The model under review builds one solid part; all positions refer to its coordinate system, in mm. A direction names the side the tool comes from. Coordinates: 2 decimals unless noted, no trailing zeros. Write each loop counter-clockwise with the first axis right and the second up, starting at its lowest first coordinate (ties: lowest second). Pieces come first, ordered by that corner, then holes. Notation, with made-up numbers: (87.5, 42.5) - (93.5, 42.5) arc R31 ccw to (93.5, 67.5) - close; hole circle Ø2 at (-38, 55). An arc over 180 degrees is marked (long way). Put each result on its own line as item: value.
from build123d import *

# Parameters (mm, degrees)
BASPROSKE_W                         = 6.35
BASPROSKE_H                         = 26.19375
TOOTHCUT_DEPTH                      = 7.35
BORSKE_R                            = 6.35
BORE_DEPTH                          = 50.8000508
SKETCH1_R                           = 23.8125
CUT_EXTRUDE1_DEPTH                  = 3.2512
F_9_64_0_14063_DIAMETER_HOLE1_D     = 3.572002
F_9_64_0_14063_DIAMETER_HOLE1_DEPTH = 9.525
F_9_64_0_14063_DIAMETER_HOLE1_TIP   = 1.073137666


with BuildPart() as part:
    # BasProSke → Base-Revolve (revolve)
    with BuildSketch(Plane(origin=(0, 0, 0), x_dir=(1, 0, 0), z_dir=(0, 1, 0))):
        with Locations((3.175, 13.096875)):
            Rectangle(BASPROSKE_W, BASPROSKE_H)
    revolve(axis=Axis((-10, 0, 0), (1, 0, 0)))

    # TooCutSke → ToothCut (cut, through all)
    with BuildSketch(Plane(origin=(0, 0, 0), x_dir=(0, 0, -1), z_dir=(1, 0, 0))):
        with BuildLine():
            ThreePointArc((0.33374141, 24.394417139), (0, 24.3967), (-0.33374141, 24.394417139))
            ThreePointArc((-0.33374141, 24.394417139), (-0.642437388, 25.31332079), (-1.03730144, 26.19862272))
            ThreePointArc((-1.03730144, 26.19862272), (0, 26.21915), (1.03730144, 26.19862272))
            ThreePointArc((1.03730144, 26.19862272), (0.642437388, 25.31332079), (0.33374141, 24.394417139))
        make_face()
    extrude(amount=TOOTHCUT_DEPTH, mode=Mode.SUBTRACT)

    # BorSke → Bore (cut, symmetric)
    with BuildSketch(Plane(origin=(0, 0, 0), x_dir=(0, 0, -1), z_dir=(1, 0, 0))):
        Circle(BORSKE_R)
    extrude(amount=BORE_DEPTH, both=True, mode=Mode.SUBTRACT)

    # Sketch1 → Cut-Extrude1 (cut)
    with BuildSketch(Plane(origin=(6.35, 0, 0), x_dir=(0, 0, -1), z_dir=(1, 0, 0))):
        Circle(SKETCH1_R)
    extrude(amount=-CUT_EXTRUDE1_DEPTH, mode=Mode.SUBTRACT)

    # 9/64 (0.14063) Diameter Hole1
    with Locations(Plane(origin=(3.0988, 0, 0), x_dir=(0, 0, -1), z_dir=(1, 0, 0))):
        with Locations((0, 9.779), (0, 19.05), (7.290119387, 17.599905094), (13.470384182, 13.470384182), (17.599905094, 7.290119387), (19.05, 0), (17.599905094, -7.290119387), (13.470384182, -13.470384182), (7.290119387, -17.599905094), (0, -19.05), (-7.290119387, -17.599905094), (-13.470384182, -13.470384182), (-17.599905094, -7.290119387), (-19.05, 0), (-17.599905094, 7.290119387), (-13.470384182, 13.470384182), (-7.290119387, 17.599905094), (6.914797213, 6.914797213), (9.779, 0), (6.914797213, -6.914797213), (0, -9.779), (-6.914797213, -6.914797213), (-9.779, 0), (-6.914797213, 6.914797213)):
            Hole(F_9_64_0_14063_DIAMETER_HOLE1_D / 2, depth=F_9_64_0_14063_DIAMETER_HOLE1_DEPTH)
            with Locations((0, 0, -(F_9_64_0_14063_DIAMETER_HOLE1_DEPTH + F_9_64_0_14063_DIAMETER_HOLE1_TIP / 2))):  # 118° drill point
                Cone(0, F_9_64_0_14063_DIAMETER_HOLE1_D / 2, F_9_64_0_14063_DIAMETER_HOLE1_TIP, mode=Mode.SUBTRACT)


solid = part.part
1. Consider section C-C on z = -10. State the section outline as (x, y) points, plus the area to 3 significant figures.
Determined:
outline: (0, -24.21) - (6.35, -24.21) - (6.35, -21.61) - (3.1, -21.61) - (3.1, -1.77) - (0, -1.77) - close; (0, 1.77) - (3.1, 1.77) - (3.1, 21.61) - (6.35, 21.61) - (6.35, 24.21) - (0, 24.21) - close
area: 156 mm^2
2. For pin 1 Ø5.5 at (y, z) = (-9.779, 0) entering from +X; pin 2 Ø3 at (x, z) = (4.5, 1) entering from -Y; pin 3 Ø1 at (x, z) = (4.5, 9) entering from -Y; pin 4 Ø4 at (y, z) = (7.29, 17.6) entering from -X, all flat-tipped, find the tip position at first contact; note any pin that passes through.
Determined:
pin 1: stops at x = 3.1
pin 2: stops at y = -26.19
pin 3: stops at y = -24.78
pin 4: stops at x = 0
3. The part is to be moulded in two halves that separate along Z. For faces 3 (the cylindrical face through (1.5, -8.4, 16.2)), 4 (the flat face through (0, -5, 5)), say which applies: +Z half, -Z half, draft (parallel to the pull), parting line (faces both ways), or undercut.
Determined:
face 3: undercut
face 4: draft
4. Consider section B-B on y = -20. State the section outline as (x, z) points.
Determined:
outline: (0, -16.91) - (6.35, -16.91) - (6.35, -12.92) - (3.1, -12.92) - (3.1, -1.51) - (0, -1.51) - close; (0, 1.51) - (3.1, 1.51) - (3.1, 12.92) - (6.35, 12.92) - (6.35, 16.91) - (0, 16.91) - close
5. Consider section D-D on z = 14.5. State the section outline as (x, y) points.
Determined:
outline: (0, -21.81) - (6.35, -21.81) - (6.35, -18.89) - (3.1, -18.89) - (3.1, -14.93) - (0, -14.93) - close; (0, -12.01) - (3.1, -12.01) - (3.1, 12.01) - (0, 12.01) - close; (0, 14.93) - (3.1, 14.93) - (3.1, 18.89) - (6.35, 18.89) - (6.35, 21.81) - (0, 21.81) - close
6. To check wall thickness, follow probe 1 along Y at (x, z) = (0.7, 0) (3 decimals); probe 2 along Y at (x, z) = (2.5, -1.5). State the ranges of each line that lie inside material, in increasing order.
Determined:
probe 1: y = -26.194 to -20.836, -17.264 to -11.565, -7.993 to -6.35, 6.35 to 7.993, 11.565 to 17.264, 20.836 to 24.397
probe 2: y = -26.15 to -20.02, -18.08 to -10.75, -8.81 to -6.17, 6.17 to 8.81, 10.75 to 18.08, 20.02 to 26.15
7. Machinability: for faces 1 (the cylindrical face through (1.53, 5.33, 7.74)), 2 (the cylindrical face through (3.131, 25.288, 0.633)), which of the approach directions +Z, -Z, +X, -X, +Y, -Y give a long, thin tool a straight path to every point of the face, cutting with its end or side? Answer none if there is none.
Determined:
face 1: +X, -X
face 2: +X, -X, +Y
8. Consider section A-A on x = 5.5. State the section outline as (y, z) points (1 decimal), plus the area to 3 significant figures.
Determined:
outline: (24.4, -0.3) arc R24.4 ccw to (24.4, 0.3) arc R10.2 ccw to (26.2, 1) arc R26.2 ccw (long way) to (26.2, -1) arc R10.2 ccw to start; hole circle Ø47.6 at (0, 0)
area: 372 mm^2
